Verification items for the finished model (mm, model axes). Round coordinates to 2 decimals unless told otherwise and drop trailing zeros. Write each loop counter-clockwise with the first axis right and the second up, starting at its lowest first coordinate (ties: lowest second). Pieces come first, ordered by that corner, then holes. Notation, with made-up numbers: M 77,42.5 L 115,42.5 A20 cw 115,50.5 Z; hole C 8.5,55.5 d8. An arc over 180 degrees is marked long. One line per item, written item: value. Start each with the question number.
Item 1: Gauge pin test, flat ends, axial feed: pin 1 (1.2 mm diameter, centred on y = -0.5, z = -18.5, fed in from -X); pin 2 (0.8 mm diameter, centred on y = 1, z = -39, fed in from -X); pin 3 (1 mm diameter, centred on x = -2.5, z = -43, fed in from +Y). Record the tip position at first contact, or that the pin passes through.
Item 2: Thickness scan on probe 1 along Z at (x, y) = (0, -1.45); probe 2 along Z at (x, y) = (-1, -0.75); probe 3 along X at (y, z) = (0.5, -32.5). Record the ranges inside material, lowest first. Write a range as from..to.
Item 3: Section check A-A, the plane z = -43. Record the cut outline in (x, y), then the cut area to 3 significant figures.
Item 4: Section check C-C, the plane z = -32.5. Record the cut outline in (x, y), then the cut area to 4 significant figures.
Item 5: Section check D-D, the plane y = 2.75. Record the cut outline in (x, z).
Item 6: Section check B-B, the plane x = 0. Record the cut outline in (y, z).
from build123d import *

# Parameters (mm, degrees)
BASE_FLANGE1_DEPTH                           = 1.5
CHAMFER1_SIZE                                = 2
CSK_FOR_M3_COUNTERSUNK_FLAT_HEAD_SCR_2_COUNT = 2
CSK_FOR_M3_COUNTERSUNK_FLAT_HEAD_SCR_2_PITCH = 18
CSK_FOR_M3_COUNTERSUNK_FLAT_HEAD_SCR_3_COUNT = 2
CSK_FOR_M3_COUNTERSUNK_FLAT_HEAD_SCR_3_PITCH = 36
SKETCHED_START                               = -50
SKETCHED_BEND1_DEPTH                         = 24.8
SKETCHED_BEND1_2_DEPTH                       = 24.8


# Read off the part's stored shape, not the designer's step: Sketched Bend1
# Sheet-metal steps are written as plain solids
with BuildPart() as part:
    # Sketch1 → Base-Flange1 (new body)
    with BuildSketch(Plane(origin=(0, 0, 0), x_dir=(1, 0, 0), z_dir=(0, 1, 0))):
        Polygon((-28.5, 50), (10, 50), (10, 0), (-10, 0), (-10, 25.2), (-28.5, 25.2), align=None)
    extrude(amount=-BASE_FLANGE1_DEPTH)

    # Chamfer1
    chamfer1_edges = [part.edges().sort_by_distance(p)[0] for p in [
        (10, -0.75, 0),
        (-10, -0.75, 0),
        (10, -0.75, -50),
    ]]
    chamfer(chamfer1_edges, length=CHAMFER1_SIZE)

    # Sketch7 → CSK for M3 Countersunk Flat Head Screw1 (revolve, cut)
    with BuildSketch(Plane(origin=(0, 0, -43), x_dir=(0, 0, 1), z_dir=(1, 0, 0))):
        Polygon((0, 0), (0, 1.5), (1.7, 1.5), (1.7, 1.45), (3.15, 0), align=None)
    csk_for_m3_countersunk_flat_head_screw1 = revolve(axis=Axis((0, 6.35, -43), (0, -1, 0)), mode=Mode.SUBTRACT)

    # CSK for M3 Countersunk Flat Head Scr 2: CSK for M3 Countersunk Flat Head Screw1 ×2
    with Locations(*[(0, 0, i * CSK_FOR_M3_COUNTERSUNK_FLAT_HEAD_SCR_2_PITCH) for i in range(1, CSK_FOR_M3_COUNTERSUNK_FLAT_HEAD_SCR_2_COUNT)]):
        add(csk_for_m3_countersunk_flat_head_screw1, mode=Mode.SUBTRACT)

    # CSK for M3 Countersunk Flat Head Scr 3: CSK for M3 Countersunk Flat Head Screw1 ×2
    with Locations(*[(0, 0, i * CSK_FOR_M3_COUNTERSUNK_FLAT_HEAD_SCR_3_PITCH) for i in range(1, CSK_FOR_M3_COUNTERSUNK_FLAT_HEAD_SCR_3_COUNT)]):
        add(csk_for_m3_countersunk_flat_head_screw1, mode=Mode.SUBTRACT)

    # Sketched Bend1 outline → Sketched Bend1 (cut)
    with BuildSketch(Plane.XY.offset(SKETCHED_START)):
        with BuildLine():
            ThreePointArc((-14, -1.5), (-15.620185175, -1.102418411), (-16.872281323, 0))
            Line((-16.872281323, 0), (-28.5, 0))
            Line((-28.5, 0), (-28.5, -1.5))
            Line((-28.5, -1.5), (-14, -1.5))
        make_face()
    extrude(amount=SKETCHED_BEND1_DEPTH, mode=Mode.SUBTRACT)

    # Sketched Bend1 2 outline → Sketched Bend1 2 (add)
    with BuildSketch(Plane.XY.offset(SKETCHED_START)):
        with BuildLine():
            Line((-10.5, 0.459069696), (-10.5, 2))
            ThreePointArc((-10.5, 2), (-15.048097173, 5.33938502), (-16.872281323, 0))
            Line((-16.872281323, 0), (-14, 0))
            ThreePointArc((-14, 0), (-15.414213562, 3.414213562), (-12, 2))
            Line((-12, 2), (-12, 0.459069696))
            Line((-12, 0.459069696), (-10.5, 0.459069696))
        make_face()
    extrude(amount=SKETCHED_BEND1_2_DEPTH)


solid = part.part
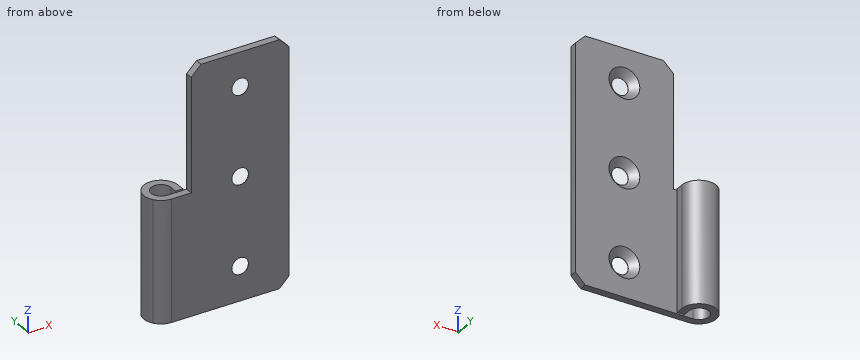
Response values:
1. pin 1: stops at x = -10
1. pin 2: stops at x = -17.45
1. pin 3: stops at y = -0.15
2. probe 1: z = -50..-44.7, -41.3..-26.7, -23.3..-8.7, -5.3..0
2. probe 2: z = -50..-45.18, -40.82..-27.18, -22.82..-9.18, -4.82..0
2. probe 3: x = -17.16..-15.32, -12..-10.5
3. outline: M -14,-1.5 L -1.7,-1.5 L -1.7,-1.45 L -3.15,0 L -14,0 A2 cw long -12,2 L -12,0.46 L -10.5,0.46 L -10.5,2 A3.5 ccw long Z; M 1.7,-1.5 L 10,-1.5 L 10,0 L 3.15,0 L 1.7,-1.45 Z
3. area: 50.5 mm2
4. outline: M -14,-1.5 L 10,-1.5 L 10,0 L -14,0 A2 cw long -12,2 L -12,0.46 L -10.5,0.46 L -10.5,2 A3.5 ccw long Z
4. area: 57.75 mm2
5. outline: M -17.42,-50 L -15.85,-50 L -15.85,-25.2 L -17.42,-25.2 Z; M -12.15,-50 L -10.58,-50 L -10.58,-25.2 L -12.15,-25.2 Z
6. outline: M -1.5,-50 L 0,-50 L 0,-46.15 L -1.45,-44.7 L -1.5,-44.7 Z; M -1.5,-41.3 L -1.45,-41.3 L 0,-39.85 L 0,-28.15 L -1.45,-26.7 L -1.5,-26.7 Z; M -1.5,-23.3 L -1.45,-23.3 L 0,-21.85 L 0,-10.15 L -1.45,-8.7 L -1.5,-8.7 Z; M -1.5,-5.3 L -1.45,-5.3 L 0,-3.85 L 0,0 L -1.5,0 Z
